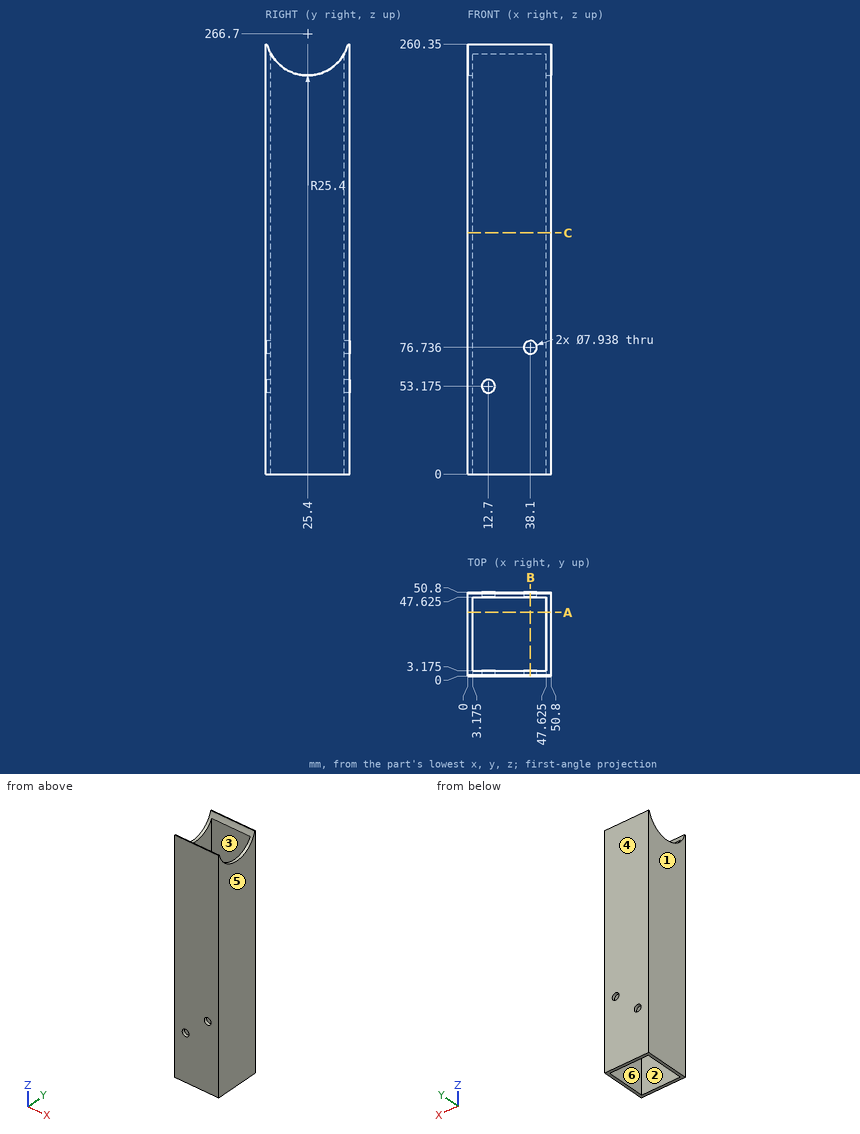
The drawing under review shows one solid part. Ordinate dimensions are in mm from its lowest x, y, z. A direction names the side the tool comes from. Coordinates: 2 decimals unless noted, no trailing zeros. Write each loop counter-clockwise with the first axis right and the second up, starting at its lowest first coordinate (ties: lowest second). Pieces come first, ordered by that corner, then holes. Notation, with made-up numbers: (8, 75.5) -> (18, 75.5) arc R22 ccw to (18, 83.5) -> close; hole circle Ø10 at (-5, 25). An arc over 180 degrees is marked (long way). One line per item, written item: value. Start each with the question number.
Q1. Add section B-B, the plane x = 38.1. Count the separate pieces of the cut face and the enclosed holes in it, then the cut area to 3 significant figures.
Q2. For the marked faces 1 and 2, list the 3-axis set-ups (+Z, -Z, +X, -X, +Y, -Y) from which the entire face can be reached by the end or side of a thin tool; tool diameter is ignored.
Q3. Add section C-C, the plane z = 146. Give the boundary of the cut face in (x, y) (1 decimal).
Q4. Clearance check with a flat-ended pin moving along its axis: P1, Ø5, axis at x = 38.1, z = 76.74, coming from the +Y side. State where the tip first meets the part, or that it passes through.
Q5. To check wall thickness, follow probe 1 along X at (y, z) = (22, 171) (1 decimal); probe 2 along Z at (x, y) = (40.5, 48) (1 decimal). State the ranges of each line that lie inside material, in increasing order.
Q6. The part is to be moulded in two halves that separate along X. For the marked faces 3, 4, 5 and 6, say which applies: +X half, -X half, draft (parallel to the pull), parting line (faces both ways), or undercut.
Q7. Add section A-A, the plane y = 38.5. Give the boundary of the cut face in (x, z) (1 decimal).
Response:
1. separate pieces: 4
1. enclosed holes: 0
1. area: 1,590 mm²
2. face 1: +Z, -Z, -X, +Y, -Y
2. face 2: +Z, -Z
3. outline: (0, 0) -> (50.8, 0) -> (50.8, 50.8) -> (0, 50.8) -> close; hole (3.2, 3.2) -> (47.6, 3.2) -> (47.6, 47.6) -> (3.2, 47.6) -> close
4. P1: through
5. probe 1: 0 to 3.2, 47.6 to 50.8
5. probe 2: 0 to 73.6, 79.9 to 255.1
6. face 3: undercut
6. face 4: draft
6. face 5: +X half
6. face 6: undercut
7. outline: (0, 0) -> (3.2, 0) -> (3.2, 244.9) -> (0, 244.9) -> close; (47.6, 0) -> (50.8, 0) -> (50.8, 244.9) -> (47.6, 244.9) -> close
